Geometry: final body of the model. Coordinates: model frame, mm. A direction names the side the tool comes from. Give positions to 0.01 mm unless a question says otherwise; leave off trailing zeros. Loops run counter-clockwise (first coordinate to the right, second up) from the corner with the lowest first, then second, coordinate; pieces in that order, holes last. Notation, with made-up numbers: (54, 35.25) - (75, 35.25) arc R21 ccw to (75, 64.25) - close; hole circle Ø2 at (10.5, -11.75). An arc over 180 degrees is marked (long way). Answer in a Markdown table with one row per item.
Autodesk Fusion 360 part; units mm, degrees
sketch "Sketch1" plane through (0, 0, 0) normal (0, 0, 1) x (1, 0, 0)
  line L0 (0, 0) -> (22.5, 0)
  line L1 (22.5, 0) -> (22.5, -22.5)
  line L2 (22.5, -22.5) -> (-22.5, -22.5)
  line L3 (-22.5, -22.5) -> (-22.5, 22.5)
  line L4 (-22.5, 22.5) -> (22.5, 22.5)
  line L5 (22.5, 22.5) -> (22.5, 0)
  circle A0 centre (0, 0) radius 12.5
  line L6 (24.5, 0) -> (24.5, -24.5)
  line L7 (24.5, -24.5) -> (-24.5, -24.5)
  line L8 (-24.5, -24.5) -> (-24.5, 24.5)
  line L9 (-24.5, 24.5) -> (24.5, 24.5)
  line L10 (24.5, 24.5) -> (24.5, 0)
  dimension "d1" = 22.5
  dimension "d2" = 22.5
  dimension "d3" = 45
  dimension "d4" = 45
  dimension "d5" = 25
  dimension "d6" = -2
extrude "Extrude1" add sketch "Sketch1" along normal blind 7 contours L1 L2 L3 L4 L5
extrude "Extrude2" add sketch "Sketch1" along normal blind 27 contours L6 L7 L8 L9 L10
sketch "Sketch2" plane through (0, 0, 0) normal (0, 0, -1) x (1, 0, 0)
  line L0 (-24.5, -24.5) -> (24.5, -24.5)
  line L1 (24.5, -24.5) -> (24.5, 24.5)
  line L2 (24.5, 24.5) -> (-24.5, 24.5)
  line L3 (-24.5, 24.5) -> (-24.5, -24.5)
  circle A0 centre (0, 0) radius 12.5
  line L4 (0, 0) -> (-29.5, 0)
  line L5 (-29.5, 0) -> (-29.5, 29.5)
  line L6 (-29.5, 29.5) -> (29.5, 29.5)
  line L7 (29.5, 29.5) -> (29.5, -29.5)
  line L8 (29.5, -29.5) -> (-29.5, -29.5)
  line L9 (-29.5, -29.5) -> (-29.5, 0)
  line L10 (-29.5, 0) -> (-40, 0)
  line L11 (29.5, 0) -> (40, 0)
  circle A1 centre (-40, 0) radius 10.75
  circle A2 centre (40, 0) radius 10.75
  line L12 (55.5, 29.5) -> (55.5, -29.5)
  line L13 (-55.5, -29.5) -> (-55.5, 0)
  line L14 (-55.5, 0) -> (-55.5, 29.5)
  line L15 (-29.5, -29.5) -> (-55.5, -29.5)
  line L16 (-55.5, 29.5) -> (-29.5, 29.5)
  line L17 (29.5, 29.5) -> (55.5, 29.5)
  line L18 (55.5, -29.5) -> (29.5, -29.5)
  dimension "d11" = 29.5
  dimension "d12" = 29.5
  dimension "d13" = 59
  dimension "d14" = 59
  dimension "d15" = 59
  dimension "d16" = 10.5
  dimension "d17" = 10.5
  dimension "d18" = 21.5
  dimension "d19" = 21.5
  dimension "d20" = -26
  dimension "d21" = -26
extrude "Extrude3" add sketch "Sketch2" against normal blind 7 contours L5 L6 L7 L8 L9 A1 A2 | L4 L9 A1 | L4 L5 A1 | L5 L9 A1 L13 L14 L15 L16 | L7 A2 L12 L17 L18 | L7 A2 picked at (29.426, 1.0262)
sketch "Sketch3" plane through (0, 0, 0) normal (0, 0, -1) x (1, 0, 0)
  line L0 (55.5, -29.5) -> (55.5, 29.5)
  line L1 (55.5, 29.5) -> (-55.5, 29.5)
  line L2 (-55.5, 29.5) -> (-55.5, -29.5)
  line L3 (-55.5, -29.5) -> (55.5, -29.5)
  circle A0 centre (40, 0) radius 10.75
  circle A1 centre (-40, 0) radius 10.75
  circle A2 centre (0, 0) radius 12.5
  line L4 (-55.5, -29.5) -> (-62.5, -29.5)
  line L5 (-55.5, 29.5) -> (-62.5, 29.5)
  line L6 (-62.5, -29.5) -> (-62.5, 29.5)
  dimension "d24" = 7
  dimension "d25" = 7
extrude "Extrude4" add sketch "Sketch3" against normal blind 80 contours L2 L4 L5 L6
sketch "Sketch4" plane through (-62.5, 0, 0) normal (-1, 0, 0) x (0, -1, 0)
  line L0 (-29.5, 0) -> (29.5, 0)
  line L1 (29.5, 0) -> (29.5, 80)
  line L2 (29.5, 80) -> (-29.5, 80)
  line L3 (-29.5, 80) -> (-29.5, 0)
  line L4 (29.5, 70.5) -> (-29.5, 70.5)
  line L5 (0, 70.5) -> (20.25, 70.5)
  line L6 (20.25, 70.5) -> (20.25, 50)
  line L7 (20.25, 50) -> (-20.25, 50)
  line L8 (-20.25, 50) -> (-20.25, 70.5)
  line L9 (-20.25, 70.5) -> (20.25, 70.5)
  line L10 (22.25, 72.5) -> (22.25, 48)
  line L11 (22.25, 48) -> (-22.25, 48)
  line L12 (-22.25, 48) -> (-22.25, 72.5)
  line L13 (-22.25, 72.5) -> (22.25, 72.5)
  dimension "d28" = -9.5
  dimension "d29" = 20.25
  dimension "d30" = 20.5
  dimension "d31" = 40.5
  dimension "d32" = -2
extrude "Extrude5" cut sketch "Sketch4" against normal blind 7 contours L4 L5 L6 L7 L8 L9
sketch "Sketch5" plane through (24.5, 0, 0) normal (1, 0, 0) x (0, 1, 0)
  line L0 (-24.5, 7) -> (24.5, 7)
  line L1 (24.5, 7) -> (24.5, 27)
  line L2 (24.5, 27) -> (-24.5, 27)
  line L3 (-24.5, 27) -> (-24.5, 7)
  circle A0 centre (0, 22) radius 1.5
  dimension "d35" = 3
  dimension "d36" = 24.5
  dimension "d37" = 15
sketch "Sketch6" plane through (0, 24.5, 0) normal (0, 1, 0) x (-1, 0, 0)
  line L0 (-24.5, 7) -> (24.5, 7)
  line L1 (24.5, 7) -> (24.5, 27)
  line L2 (24.5, 27) -> (-24.5, 27)
  line L3 (-24.5, 27) -> (-24.5, 7)
  circle A0 centre (0, 22) radius 1.5
  dimension "d38" = 3
  dimension "d39" = 24.5
  dimension "d40" = 15
extrude "Extrude6" cut sketch "Sketch5" against normal blind 55 contours A0
extrude "Extrude7" cut sketch "Sketch6" against normal blind 55 contours A0
Q1. Cut plane A-A (x = 40). Output: boundary loops of the cut face in (y, z), and give its area (4 significant figures).
Check values:
| item | result |
|---|---|
| outline | (-29.5, 0) - (-10.75, 0) - (-10.75, 7) - (-29.5, 7) - close; (10.75, 0) - (29.5, 0) - (29.5, 7) - (10.75, 7) - close |
| area | 262.5 mm² |
Q2. Cut plane C-C (x = 0). Output: boundary loops of the cut face in (y, z).
Check values:
| item | result |
|---|---|
| outline | (-29.5, 0) - (-12.5, 0) - (-12.5, 7) - (-22.5, 7) - (-22.5, 20.5) - (-24.5, 20.5) - (-24.5, 7) - (-29.5, 7) - close; (-24.5, 23.5) - (-22.5, 23.5) - (-22.5, 27) - (-24.5, 27) - close; (12.5, 0) - (29.5, 0) - (29.5, 7) - (24.5, 7) - (24.5, 20.5) - (22.5, 20.5) - (22.5, 7) - (12.5, 7) - close; (22.5, 23.5) - (24.5, 23.5) - (24.5, 27) - (22.5, 27) - close |
Q3. Reachability of faces 1 (the flat face through (0, 24.5, 17)), 2 (the flat face through (-59, 20.25, 60)), 3 (the flat face through (24.5, 0, 17)), 4 (the flat face through (-29.5, 0, 3)), 5 (the flat face through (0, -22.5, 17)) from +Z, -Z, +X, -X, +Y, -Y: full face, straight path, thin tool, end or side. Return the list, or none.
Check values:
| item | result |
|---|---|
| face 1 | +Z, +X, +Y |
| face 2 | +X, -X |
| face 3 | +Z, +X, +Y, -Y |
| face 4 | +Z, -Z |
| face 5 | +Z |
Q4. Cut plane B-B (z = 22). Output: boundary loops of the cut face in (x, y), and give its area (3 significant figures).
Check values:
| item | result |
|---|---|
| outline | (-62.5, -29.5) - (-55.5, -29.5) - (-55.5, 29.5) - (-62.5, 29.5) - close; (-24.5, -24.5) - (-1.5, -24.5) - (-1.5, -22.5) - (-22.5, -22.5) - (-22.5, -1.5) - (-24.5, -1.5) - close; (-24.5, 1.5) - (-22.5, 1.5) - (-22.5, 22.5) - (-1.5, 22.5) - (-1.5, 24.5) - (-24.5, 24.5) - close; (1.5, -24.5) - (24.5, -24.5) - (24.5, -1.5) - (22.5, -1.5) - (22.5, -22.5) - (1.5, -22.5) - close; (1.5, 22.5) - (22.5, 22.5) - (22.5, 1.5) - (24.5, 1.5) - (24.5, 24.5) - (1.5, 24.5) - close |
| area | 765 mm² |
Q5. Cut plane D-D (z = 58). Output: boundary loops of the cut face in (x, y), and give its area (4 significant figures).
Check values:
| item | result |
|---|---|
| outline | (-62.5, -29.5) - (-55.5, -29.5) - (-55.5, -20.25) - (-62.5, -20.25) - close; (-62.5, 20.25) - (-55.5, 20.25) - (-55.5, 29.5) - (-62.5, 29.5) - close |
| area | 129.5 mm² |
Q6. First-contact query: pin 1 (8 mm diameter, centred on y = -10, z = 23.5, fed in from +X); pin 2 (1.5 mm diameter, centred on y = -21.5, z = 62, fed in from +X); pin 3 (10 mm diameter, centred on x = -10, z = 14, fed in from +Y). Flat tips, straight axial feed; report the tip coordinate or a pass-through.
Check values:
| item | result |
|---|---|
| pin 1 | x = 24.5 |
| pin 2 | x = -55.5 |
| pin 3 | y = 24.5 |
Q7. Draft query along Z for faces 6 (the flat face through (-59, -20.25, 60)), 7 (the flat face through (-59, 0, 70.5)), 8 (the flat face through (-24.5, 0, 17)), 9 (the flat face through (-17, 0, 0)). Return one class per face: pulls with the +Z half, pulls with the -Z half, needs draft (parallel to the pull), parting line crosses it, or undercut.
Check values:
| item | result |
|---|---|
| face 6 | undercut |
| face 7 | undercut |
| face 8 | needs draft |
| face 9 | pulls with the -Z half |
Q8. Material intervals for line 1 along X through (y, z) = (3, 13); line 2 along Y through (x, z) = (-40, 3); line 3 along Y through (x, z) = (0, 3.5), sorted ascending.
Check values:
| item | result |
|---|---|
| line 1 | -62.5 to -55.5, -24.5 to -22.5, 22.5 to 24.5 |
| line 2 | -29.5 to -10.75, 10.75 to 29.5 |
| line 3 | -29.5 to -12.5, 12.5 to 29.5 |
